The model under review builds one solid part; all positions refer to its coordinate system, in mm. Face numbers are marked on the shaded views. Round coordinates to 2 decimals unless told otherwise and drop trailing zeros. Order: outer loops, then holes, each group sorted by start corner. A loop starts at its lowest first (then second) coordinate and runs counter-clockwise, first axis right, second up. Notation, with made-up numbers: M -11.75,51.5 L 0.25,51.5 A19 cw 0.25,81.5 Z; hole C -5.75,-29 d11. An arc over 180 degrees is marked long. Answer as a JSON object with one key per item and string values. Group by question number.
1) To check wall thickness, follow line 1 (Z direction, x = 33, y = 28); line 2 (X direction, y = 35.5, z = 17.5); line 3 (Z direction, x = 18, y = 9.5). State the ranges of each line that lie inside material, in increasing order.
2) Consider section B-B, the plane y = 8. Count the separate pieces of the cut face and the enclosed holes in it, then the cut area to 3 significant figures.
3) Insertion check: pin 1 Ø11 at (x, z) = (29.14, 16.94) entering from -Y; pin 2 Ø6 at (y, z) = (31.5, -25) entering from +X; pin 3 Ø12.5 at (x, z) = (17.89, -18.35) entering from -Y. Each pin has a flat end and moves straight along its axis. Give the tip position at first contact, or say it passes through.
4) Consider section D-D, the plane z = 34. Write out the cut boundary in (x, y), then the cut area to 3 significant figures.
5) Consider section C-C, the plane x = -43. Write out the cut boundary in (y, z).
6) Consider section A-A, the plane z = 15.5. Write out the cut boundary in (x, y), then the cut area to 3 significant figures.
7) The part is to be moulded in two halves that separate along X. For the marked faces 1, 2, 3 and 4, say which applies: +X half, -X half, draft (parallel to the pull), parting line (faces both ways), or undercut.
```python
from build123d import *

# Parameters (mm, degrees)
F0_R           = 50.8
F0_R_2         = 1.5875
F0_R_3         = 9.525
F0_R_4         = 5.715
F0_R_5         = 3.175
F0_R_6         = 4.7625
F1_DEPTH       = 38.1
F2_D           = 6.35
F3_D           = 9.525
F3_CBORE_D     = 19.05
F3_CBORE_DEPTH = 6.35
F4_D           = 9.525
F4_CSINK_D     = 19.05
F4_CSINK_ANGLE = 82
F5_D           = 5.1054
F5_DEPTH       = 38.1
F5_TIP         = 1.5338169022
F6_D           = 11.43


with BuildPart() as f1:
    # F0 (on Front) → F1 (new body)
    with BuildSketch(Plane.XZ):
        with Locations((-1.0572489118, 7.1283597499)):
            Circle(F0_R)
        with Locations((-20.0026774298, -18.3497335514)):
            Circle(F0_R_2, mode=Mode.SUBTRACT)
        with Locations((17.8881796061, -18.3497335514)):
            Circle(F0_R_3, mode=Mode.SUBTRACT)
        with Locations((-31.2532933042, 16.9396493213)):
            Circle(F0_R_4, mode=Mode.SUBTRACT)
        with Locations((-1.0572489118, 38.8783597499)):
            Circle(F0_R_5, mode=Mode.SUBTRACT)
        with Locations((29.1387954806, 16.9396493213)):
            Circle(F0_R_3, mode=Mode.SUBTRACT)
        with Locations((29.1387954806, 16.9396493213)):
            Circle(F0_R_3)
        with Locations((29.1387954806, 16.9396493213)):
            Circle(F0_R_6, mode=Mode.SUBTRACT)
        with Locations((17.8881796061, -18.3497335514)):
            Circle(F0_R_3)
        with Locations((17.8881796061, -18.3497335514)):
            Circle(F0_R_6, mode=Mode.SUBTRACT)
        with Locations((-31.2532933042, 16.9396493213)):
            Circle(F0_R_4)
        with Locations((29.1387954806, 16.9396493213)):
            Circle(F0_R_6)
        with Locations((17.8881796061, -18.3497335514)):
            Circle(F0_R_6)
        with Locations((-1.0572489118, 38.8783597499)):
            Circle(F0_R_5)
        with Locations((-20.0026774298, -18.3497335514)):
            Circle(F0_R_2)
    extrude(amount=-F1_DEPTH)

    # F2 (through all)
    with Locations(Plane.XZ):
        with Locations((-1.0572489118, 38.8783597499)):
            Hole(F2_D / 2)

    # F3 (through all)
    with Locations(Plane.XZ):
        with Locations((29.1387954806, 16.9396493213)):
            CounterBoreHole(F3_D / 2, F3_CBORE_D / 2, F3_CBORE_DEPTH)

    # F4 (through all)
    with Locations(Plane.XZ):
        with Locations((17.8881796061, -18.3497335514)):
            CounterSinkHole(F4_D / 2, F4_CSINK_D / 2, counter_sink_angle=F4_CSINK_ANGLE)

    # F5
    with Locations(Plane.XZ):
        with Locations((-20.0026774298, -18.3497335514)):
            Hole(F5_D / 2, depth=F5_DEPTH)
            with Locations((0, 0, -(F5_DEPTH + F5_TIP / 2))):  # 118° drill point
                Cone(0, F5_D / 2, F5_TIP, mode=Mode.SUBTRACT)

    # F6 (through all)
    with Locations(Plane.XZ):
        with Locations((-31.2532933042, 16.9396493213)):
            Hole(F6_D / 2)


solid = f1.part
```
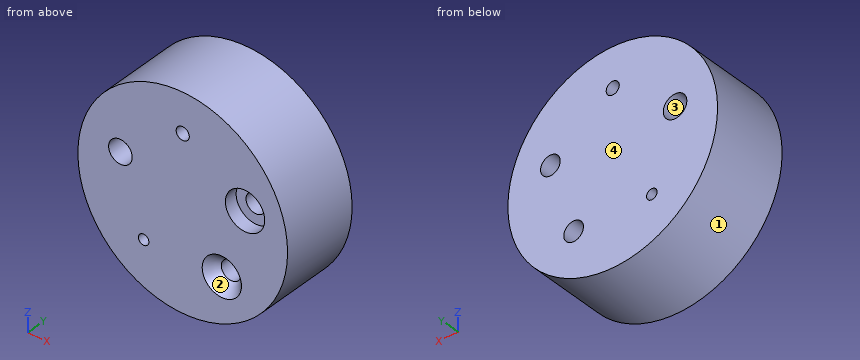
Results list:
{
 "1": {"line 1": "-30.56 to 14.15, 19.73 to 44.82", "line 2": "-50.79 to -36.94, -25.57 to 24.41, 33.87 to 48.67", "line 3": "-39.96 to -23.11, -13.59 to 54.22"},
 "2": {"separate pieces": "1", "enclosed holes": "5", "area": "7,810 mm^2"},
 "3": {"pin 1": "y = 6.35", "pin 2": "x = 40.56", "pin 3": "y = 3.77"},
 "4": {"outline": "M -44.17,0 L 42.05,0 L 42.05,38.1 L -44.17,38.1 Z", "area": "3,290 mm^2"},
 "5": {"outline": "M 0,-21.53 L 38.1,-21.53 L 38.1,35.79 L 0,35.79 Z"},
 "6": {"outline": "M -51.16,0 L -36.78,0 L -36.78,38.1 L -51.16,38.1 Z; M -25.72,0 L 19.72,0 L 19.72,6.35 L 24.6,6.35 L 24.6,38.1 L -25.72,38.1 Z; M 33.68,6.35 L 38.55,6.35 L 38.55,0 L 49.05,0 L 49.05,38.1 L 33.68,38.1 Z", "area": "2,990 mm^2"},
 "7": {"face 1": "parting line", "face 2": "undercut", "face 3": "undercut", "face 4": "draft"}
}
